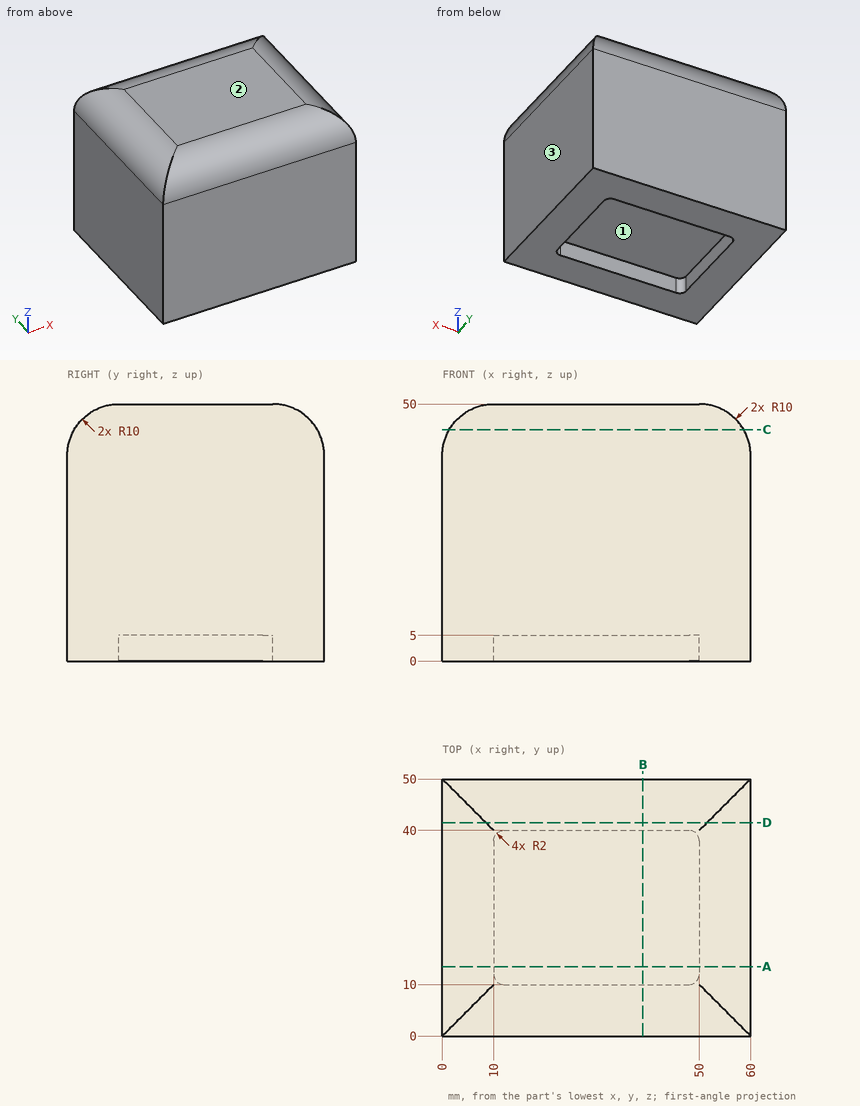
Drawing for the job (mm, zero at the part's lowest x, y, z). Round coordinates to 2 decimals unless told otherwise and drop trailing zeros. Order: outer loops, then holes, each group sorted by start corner. A loop starts at its lowest first (then second) coordinate and runs counter-clockwise, first axis right, second up. Notation, with made-up numbers: (26.5, 31.25) -> (77.5, 31.25) arc R12 ccw to (77.5, 49.25) -> close; hole circle Ø11 at (23, -17). An arc over 180 degrees is marked (long way). Put each result on its own line as item: value.
Q1. Band-saw the part on A-A (y = 13.5). Give the cut face in (x, z).
From the geometry:
outline: (0, 0) -> (10, 0) -> (10, 5) -> (50, 5) -> (50, 0) -> (60, 0) -> (60, 40) arc R10 ccw to (50, 50) -> (10, 50) arc R10 ccw to (0, 40) -> close
Q2. Band-saw the part on D-D (y = 41.5). Give the cut face in (x, z), and give its area (3 significant figures).
From the geometry:
outline: (0, 0) -> (60, 0) -> (60, 40) arc R10 ccw to (51.5, 49.89) -> (8.5, 49.89) arc R10 ccw to (0, 40) -> close
area: 2,950 mm2
Q3. Pull direction X, two halves, no side cores. Call the marked faces 1, 2 and 3: pulls with the +X half, pulls with the -X half, needs draft (parallel to the pull), parting line crosses it, or undercut.
From the geometry:
face 1: undercut
face 2: needs draft
face 3: pulls with the +X half
Q4. Pin check, flat tip, straight feed: pin 1 Ø15 at (x, y) = (32, 24) entering from -Z. Stop position of the tip, or through.
From the geometry:
pin 1: stops at z = 5
Q5. Band-saw the part on C-C (z = 45). Give the cut face in (x, y), and give its area (3 significant figures).
From the geometry:
outline: (1.34, 1.34) -> (58.66, 1.34) -> (58.66, 48.66) -> (1.34, 48.66) -> close
area: 2,710 mm2
Q6. Band-saw the part on B-B (x = 39). Give the cut face in (y, z).
From the geometry:
outline: (0, 0) -> (10, 0) -> (10, 5) -> (40, 5) -> (40, 0) -> (50, 0) -> (50, 40) arc R10 ccw to (40, 50) -> (10, 50) arc R10 ccw to (0, 40) -> close
Q7. Wall check: line 1 (X direction, y = 28.5, z = 3); line 2 (Z direction, x = 28, y = 18); line 3 (Z direction, x = 55.5, y = 41.5). Give the ranges that are in metal, low to high. Write a range as [from, to].
From the geometry:
line 1: x = [0, 10], [50, 60]
line 2: z = [5, 50]
line 3: z = [0, 48.35]
